Check sheet for the modelled part. Datum: model origin and axes. Units: mm. Round coordinates to 2 decimals unless told otherwise and drop trailing zeros. Write each loop counter-clockwise with the first axis right and the second up, starting at its lowest first coordinate (ties: lowest second). Pieces come first, ordered by that corner, then holes. Notation, with made-up numbers: (16.25, 80) -> (58.25, 80) arc R17 cw to (58.25, 89) -> close; hole circle Ø10 at (-21, 72.5). An arc over 180 degrees is marked (long way). Write item = value, one per line.
from build123d import *

# Parameters (mm, degrees)
F0_W     = 136.742865
F0_H     = 90.413568
F0_R     = 19.05
F1_DEPTH = 50.8


with BuildPart() as f1:
    # F0 (on Top) → F1 (new body)
    with BuildSketch(Plane.XY):
        with Locations((2.551172, 0.510237)):
            Rectangle(F0_W, F0_H)
        Circle(F0_R, mode=Mode.SUBTRACT)
    extrude(amount=-F1_DEPTH)


solid = f1.part
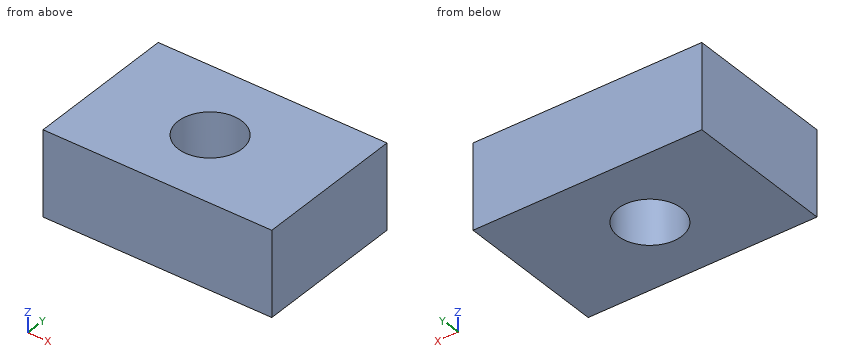
(1) Material ranges on L1, parallel to Y at x = 0, z = -22; L2, parallel to X at y = 13.5, z = -46; L3, parallel to X at y = -8.5, z = -8, recorded low to high. Write a range as [from, to].
Worked answers:
L1 = [-44.7, -19.05], [19.05, 45.72]
L2 = [-65.82, -13.44], [13.44, 70.92]
L3 = [-65.82, -17.05], [17.05, 70.92]
(2) Sectioned sample at C-C on z = -26.5. Enter the section's corners in (x, y).
Worked answers:
outline = (-65.82, -44.7) -> (70.92, -44.7) -> (70.92, 45.72) -> (-65.82, 45.72) -> close; hole circle Ø38.1 at (0, 0)
(3) Sectioned sample at A-A on x = 0. Enter the section's corners in (y, z).
Worked answers:
outline = (-44.7, -50.8) -> (-19.05, -50.8) -> (-19.05, 0) -> (-44.7, 0) -> close; (19.05, -50.8) -> (45.72, -50.8) -> (45.72, 0) -> (19.05, 0) -> close
(4) Sectioned sample at B-B on y = 0. Enter the section's corners in (x, z).
Worked answers:
outline = (-65.82, -50.8) -> (-19.05, -50.8) -> (-19.05, 0) -> (-65.82, 0) -> close; (19.05, -50.8) -> (70.92, -50.8) -> (70.92, 0) -> (19.05, 0) -> close
